Can you work these out from the model? Positions are in its coordinate system, mm. Coordinates: 2 decimals unless noted, no trailing zeros. Write each loop counter-clockwise with the first axis right and the second up, starting at its lowest first coordinate (ties: lowest second). Pieces come first, ordered by that corner, then holes. Notation, with made-up numbers: (-10.5, -19) - (37.5, -19) arc R6 ccw to (37.5, -12) - close; hole circle Ø4 at (-30, -32). An arc over 180 degrees is marked (long way). Use one line per item in the form item = value. Start each with the question number.
(1) For pin 1 Ø1 at (x, y) = (1, -4) entering from +Z, with a flat end and sliding along its axis, tell me the tip position at first contact or that it passes through.
(2) If we section it at B-B on x = 3.45: Please give me the cut outline in (y, z).
(3) If I drill on probe 1 along Z at (x, y) = (3.75, 0); probe 2 along Z at (x, y) = (4.55, -1.75); probe 3 along Y at (x, z) = (1.75, 2), over which ranges is the centre line in solid material (lowest first)? Write a range as from..to.
(4) If we section it at A-A on y = 0: Please give me the cut outline in (x, z).
Autodesk Inventor part; units mm, degrees
ref_plane "Work Plane1" through (-11.0799, 0, 0) normal (0, -0.8660254, -0.5) x (1, 0, 0)
ref_plane "YZ Plane" through (0, 0, 0) normal (1, 0, 0) x (0, 1, 0)
ref_plane "XZ Plane" through (0, 0, 0) normal (0, 1, 0) x (-1, 0, 0)
sketch "Sketch1" plane through (0, 0, 0) normal (1, 0, 0) x (0, 1, 0)
  line L0 (-5.7735, 0) -> (-2.8868, 5)
  line L1 (-2.8868, 5) -> (2.8868, 5)
  line L2 (2.8868, 5) -> (5.7735, 0)
  line L3 (5.7735, 0) -> (2.8868, -5)
  line L4 (2.8868, -5) -> (-2.8868, -5)
  line L5 (-2.8868, -5) -> (-5.7735, 0)
  point P0 (0, 0)
  point P1 (0, 0)
  dimension "d0" = 11.547
extrude "Body" add sketch "Sketch1" along normal blind 5
sketch "Sketch2" plane through (0, 0, 0) normal (0, 0, 1) x (1, 0, 0)
  line L0 (0, 2.8868) -> (0, 5.7735)
  line L1 (0, 5.7735) -> (5, 5.7735)
  line L2 (5, 2.8868) -> (5, 5.7735)
  line L3 (-1, 0) -> (6, 0)
  line L4 (0.8219, 5.7735) -> (0, 4.35)
  line L5 (4.1781, 5.7735) -> (5, 4.35)
  dimension "d3" = 30
  dimension "d4" = 30
  dimension "d5" = 8.7
  dimension "d6" = 8.7
revolve "Chamfer1" cut sketch "Sketch2" angle 360 about axis through (-10, 0, 0) along (1, 0, 0)
sketch "Sketch3" plane through (5, 0, 0) normal (1, 0, 0) x (0, 0, -1)
  arc A0 (-0.625, -1.0825) -> (0.625, -1.0825) centre (0, 0) ccw
hole "Thread" at (5, 0, 0) direction (-1, 0, 0) diameter 4.917 end through all
chamfer "Chamfer2" distance 0.5413 angle 30 1 edges at (5, 0, 2.4585) measured on face at (5, 3.6714, -0.4458)
chamfer "Chamfer3" distance 0.5413 angle 30 1 edges at (0, 0, 2.4585) measured on face at (0, 3.6714, -0.4458)
ref_plane "Work Plane1" through (-11.0799, 0, 0) normal (0, -0.8660254, -0.5) x (1, 0, 0)
equation "\"d0\" = 1.1547 * SW"
equation "\"d1\" = KOH"
equation "\"d3\" = ANG1"
equation "\"d4\" = ANG2"
equation "\"d5\" = SW0"
equation "\"d6\" = SW01"
equation "\"d8\" = -0.5 * GD1 + 0.5 * NND"
equation "\"d40\" = -0.5 * GD1 + 0.5 * NND"
equation "\"d10\" = -0.5 * GD1 + 0.5 * NND"
equation "\"d41\" = -0.5 * GD1 + 0.5 * NND"
equation "\"ANG1\" = 30deg"
equation "\"ANG2\" = 30deg"
equation "\"NND\" = 6"
equation "\"KOH\" = 5"
equation "\"SW0\" = 8.7"
equation "\"SW01\" = 8.7"
equation "\"GUL\" = 0.541266 * PTC"
equation "\"THREADDIA\" = 6"
equation "\"TOA\" = 30deg"
equation "\"PTC\" = 1"
equation "\"E0\" = 1.155 * SW"
equation "\"GAL\" = 0.541266 * PTC"
properties part number "DIN 555-5 - M6" material "Steel, Mild"
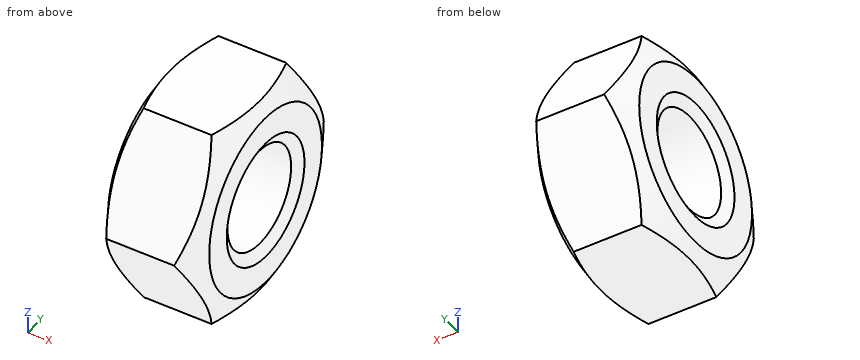
Reported:
q1.pin_1 = 3.94
q2.outline = (-5.77, 0) - (-2.89, -5) - (2.89, -5) - (5.77, 0) - (2.89, 5) - (-2.89, 5) - close; hole circle Ø4.92 at (0, 0)
q3.probe_1 = -5..-2.46, 2.46..5
q3.probe_2 = -4.82..-1.73, 1.73..4.82
q3.probe_3 = -4.62..-1.43, 1.43..4.62
q4.outline = (0, -4.35) - (0.38, -5) - (4.62, -5) - (5, -4.35) - (5, -3) - (4.69, -2.46) - (0.31, -2.46) - (0, -3) - close; (0, 3) - (0.31, 2.46) - (4.69, 2.46) - (5, 3) - (5, 4.35) - (4.62, 5) - (0.38, 5) - (0, 4.35) - close
